Can you work these out from the drawing? Everything is in mm from the part's minimum corner. A direction names the side the tool comes from. Coordinates: 2 decimals unless noted, no trailing zeros. Write each loop counter-clockwise with the first axis right and the second up, starting at its lowest first coordinate (ties: lowest second). Pieces come first, ordered by that corner, then holes.
(1) Imagine slicing it at D-D, the plane x = 24. List the corners of the cut face in (y, z) for me.
(2) Please list where these lines run through material, in increasing order: probe 1 along X at (y, z) = (6, 4.5) (1 decimal); probe 2 along X at (y, z) = (37, 2.75) (1 decimal); probe 3 along Y at (x, z) = (11, 1.75).
(3) Which directions (+Z, -Z, +X, -X, +Y, -Y) give clear straight access to the entire face, cutting with the end or side of a thin tool? Please do the marked faces 1 and 2.
(4) For pin 1 Ø3 at (x, z) = (13, 2) entering from -Y; pin 2 Ø8 at (x, y) = (18.5, 35) entering from +Z, each with a flat end and sliding along its axis, tell me the tip position at first contact or that it passes through.
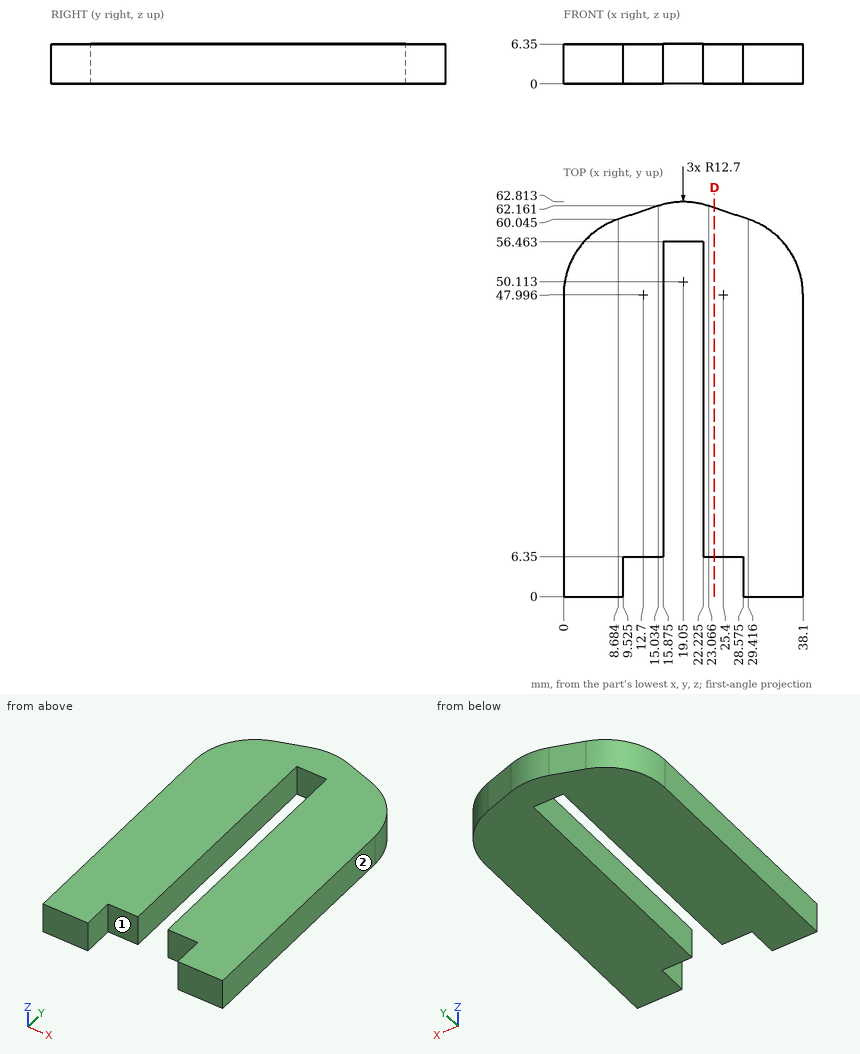
Recorded:
1. outline: (6.35, 0) - (61.85, 0) - (61.85, 6.35) - (6.35, 6.35) - close
2. probe 1: x = 0 to 9.5, 28.6 to 38.1
2. probe 2: x = 0 to 15.9, 22.2 to 38.1
2. probe 3: y = 6.35 to 60.82
3. face 1: +Z, -Z, -Y
3. face 2: +Z, -Z, +X, +Y, -Y
4. pin 1: stops at y = 6.35
4. pin 2: stops at z = 6.35
